Source: CAD feature listing. Evaluate the final solid. Frame: model axes, mm. A direction names the side the tool comes from. Coordinates: 2 decimals unless noted, no trailing zeros. Write each loop counter-clockwise with the first axis right and the second up, starting at its lowest first coordinate (ties: lowest second). Pieces come first, ordered by that corner, then holes. Notation, with made-up numbers: (41, -8) -> (69, -8) arc R24 cw to (69, 26) -> close; hole circle Ø4 at (-36.75, -35.75). An arc over 180 degrees is marked (long way). Write item = value, one per line.
from build123d import *

# Parameters (mm, degrees)
F0_R     = 25.1778110622
F0_W     = 9.7031409531
F0_H     = 27.7212755755
F1_DEPTH = 233.172
F3_DEPTH = 233.172
F4_SIZE  = 10.16
F5_R     = 2
F6_R     = 31.5278110622
F7_DEPTH = 5.08
F8_R     = 31.5278110622
F9_DEPTH = 5.08


with BuildPart() as f1:
    # F0 (on Top) → F1 (new body)
    with BuildSketch(Plane.XY):
        Polygon((-28.9911830187, 45.647662133), (-62.8567745299, 45.647662133), (-62.8567745299, -13.4259527549), (-62.8567745299, -41.1472283304), (62.8567745299, -41.1472283304), (62.8567745299, -13.4259527549), (62.8567745299, 45.647662133), (28.9911830187, 45.647662133), (0, 45.647662133), align=None)
        Circle(F0_R, mode=Mode.SUBTRACT)
        Polygon((-28.9911830187, 63.7326575816), (-28.9911830187, 45.647662133), (0, 45.647662133), (28.9911830187, 45.647662133), (28.9911830187, 63.7326575816), align=None)
        with Locations((-67.7083450064, -27.2865905426)):
            Rectangle(F0_W, F0_H)
        with Locations((67.7083450064, -27.2865905426)):
            Rectangle(F0_W, F0_H)
    extrude(amount=F1_DEPTH)

    # F2 (on face) → F3 (cut, through all)
    with BuildSketch(Plane.XY.offset(233.172)):
        Polygon((-31.8065583706, -37.138659507), (-31.8065583706, -41.1472283304), (31.8065583706, -41.1472283304), (31.8065583706, -37.138659507), (0, -37.138659507), align=None)
    extrude(amount=-F3_DEPTH, mode=Mode.SUBTRACT)

    # F4
    f4_edges = [f1.edges().sort_by_distance(p)[0] for p in [
        (-28.991183, 63.732658, 116.586),
        (28.991183, 63.732658, 116.586),
    ]]
    chamfer(f4_edges, length=F4_SIZE)

    # F5
    f5_edges = [f1.edges().sort_by_distance(p)[0] for p in [
        (72.559915, -13.425953, 116.586),
        (72.559915, -41.147228, 116.586),
        (31.806558, -41.147228, 116.586),
        (-31.806558, -41.147228, 116.586),
        (-72.559915, -41.147228, 116.586),
        (-72.559915, -13.425953, 116.586),
        (-62.856775, 45.647662, 116.586),
        (62.856775, 45.647662, 116.586),
        (62.856775, -13.425953, 116.586),
        (-62.856775, -13.425953, 116.586),
    ]]
    fillet(f5_edges, radius=F5_R)

    # F6 (on face) → F7 (cut)
    with BuildSketch(Plane(origin=(0, 0, 0), x_dir=(1, 0, 0), z_dir=(0, 0, -1))):
        Circle(F6_R)
    extrude(amount=-F7_DEPTH, mode=Mode.SUBTRACT)

    # F8 (on face) → F9 (cut)
    with BuildSketch(Plane.XY.offset(233.172)):
        Circle(F8_R)
    extrude(amount=-F9_DEPTH, mode=Mode.SUBTRACT)


solid = f1.part
1) Reachability of faces 5 (the flat face through (-28.991, 50, 115)), 6 (the flat face through (-21.2, -13.9, 228.092)), 7 (the flat face through (28.991, 50, 115)) from +Z, -Z, +X, -X, +Y, -Y: full face, straight path, thin tool, end or side. Return the list, or none.
Answer block:
face_5 = +Z, -Z, -X, +Y
face_6 = +Z
face_7 = +Z, -Z, +X, +Y
2) Cut plane B-B, the plane x = 0. Output: boundary loops of the cut face in (y, z).
Answer block:
outline = (-37.14, 0) -> (-31.53, 0) -> (-31.53, 5.08) -> (-25.18, 5.08) -> (-25.18, 228.09) -> (-31.53, 228.09) -> (-31.53, 233.17) -> (-37.14, 233.17) -> close; (25.18, 5.08) -> (31.53, 5.08) -> (31.53, 0) -> (63.73, 0) -> (63.73, 233.17) -> (31.53, 233.17) -> (31.53, 228.09) -> (25.18, 228.09) -> close
3) First-contact query: pin 1 Ø3 at (x, z) = (68.5, 61.5) entering from +Y; pin 2 Ø9.5 at (x, z) = (50.5, 91) entering from +Y; pin 3 Ø12 at (y, z) = (48, 180) entering from +X. Flat tips, straight axial feed; report the tip coordinate or a pass-through.
Answer block:
pin_1 = -13.43
pin_2 = 45.65
pin_3 = 62.86
4) Cut plane C-C, the plane y = 0. Output: boundary loops of the cut face in (x, z), and give its area (3 significant figures).
Answer block:
outline = (-62.86, 0) -> (-31.53, 0) -> (-31.53, 5.08) -> (-25.18, 5.08) -> (-25.18, 228.09) -> (-31.53, 228.09) -> (-31.53, 233.17) -> (-62.86, 233.17) -> close; (25.18, 5.08) -> (31.53, 5.08) -> (31.53, 0) -> (62.86, 0) -> (62.86, 233.17) -> (31.53, 233.17) -> (31.53, 228.09) -> (25.18, 228.09) -> close
area = 17,400 mm2
5) Pull-direction query (Y, two-part tool) for faces 1 (the flat face through (52, -41.147, 115)), 2 (the flat face through (23.982, 58.582, 114.954)), 3 (the flat face through (-72.56, -27, 115)), 4 (the flat face through (-21.2, 13.9, 5.08)); classes: +Y half, -Y half, draft (parallel to the pull), parting line (faces both ways), or undercut.
Answer block:
face_1 = -Y half
face_2 = +Y half
face_3 = draft
face_4 = undercut
6) Cut plane D-D, the plane x = 38.5. Output: boundary loops of the cut face in (y, z).
Answer block:
outline = (-41.15, 0) -> (45.65, 0) -> (45.65, 233.17) -> (-41.15, 233.17) -> close
7) Material intervals for probe 1 along X at (y, z) = (0, 3.15); probe 2 along X at (y, z) = (0, 57); probe 3 along Y at (x, z) = (0, 231.4), sorted ascending. Write a range as [from, to].
Answer block:
probe_1 = [-62.86, -31.53], [31.53, 62.86]
probe_2 = [-62.86, -25.18], [25.18, 62.86]
probe_3 = [-37.14, -31.53], [31.53, 63.73]
